```python
from build123d import *

# Parameters (mm, degrees)
BOX_W               = 29
BOX_H               = 73
BOX_DEPTH           = 10
BOX_PLACEMENT_ANGLE = 13
PAD_DEPTH           = 27.6


with BuildPart() as cube:
    # Box → Box (new body)
    with BuildSketch(Plane.XY):
        with Locations((14.5, 36.5)):
            Rectangle(BOX_W, BOX_H)
    extrude(amount=BOX_DEPTH)


with BuildPart() as cube_1:
    # Box placement: moved
    add(cube.part.moved(Location((46, -5, -10))).rotate(Axis((46, -5, -10), (0, -1, 0)), BOX_PLACEMENT_ANGLE))


with BuildPart() as cutted_flask:
    # Sketch → Pad (new body)
    with BuildSketch(Plane.XY):
        with BuildLine():
            ThreePointArc((2.776495, 50.1), (0.813217, 49.286783), (0, 47.323505))
            Line((0, 2.776495), (0, 47.323505))
            ThreePointArc((0, 2.776495), (0.813217, 0.813217), (2.776495, 0))
            Line((45.947206, 0), (2.776495, 0))
            ThreePointArc((45.947206, 0), (47.381198, 0.172613), (48.733265, 0.680592))
            Line((71.324311, 12.41834), (48.733265, 0.680592))
            ThreePointArc((71.324311, 12.41834), (71.817845, 12.880043), (72, 13.530861))
            Line((72, 25.05), (72, 13.530861))
            Line((72, 25.05), (72, 36.102443))
            ThreePointArc((72, 36.102443), (71.822776, 36.745073), (71.341206, 37.206021))
            Line((71.341206, 37.206021), (48.765787, 49.376307))
            ThreePointArc((48.765787, 49.376307), (47.376999, 49.916284), (45.898298, 50.1))
            Line((2.776495, 50.1), (45.898298, 50.1))
        make_face()
    extrude(amount=PAD_DEPTH)

    # Cut: cut Cube
    add(cube_1.part, mode=Mode.SUBTRACT)


solid = cutted_flask.part
```
Could you check a few things on this model? Use its own coordinates, in mm. Round coordinates to 2 decimals unless told otherwise and drop trailing zeros. Loops run counter-clockwise (first coordinate to the right, second up) from the corner with the lowest first, then second, coordinate; pieces in that order, holes last. Notation, with made-up numbers: (69.5, 27) - (101.5, 27) arc R24 ccw to (101.5, 64) - close; hole circle Ø5 at (0, 15). An arc over 180 degrees is marked (long way). Answer in a Markdown table with one row per item. Add a question column.
(1) If we section it at A-A (z = 25.5): Please give me the cut outline in (x, y), plus the area to 3 significant figures.
(2) I need wall thicknesses on line 1 along Y through (x, z) = (46, 22.5); line 2 along Y through (x, z) = (48.5, 11.75); line 3 along Z through (x, y) = (45, 13). Which ranges of each line are inside material? Lowest first, please.
(3) If we section it at D-D (y = 10): Please give me the cut outline in (x, z).
(4) If we section it at C-C (x = 67): Please give me the cut outline in (y, z), plus the area to 3 significant figures.
(5) If we section it at B-B (y = 33): Please give me the cut outline in (x, z).
(6) I'm going to push flat-ended pins straight in: pin 1 (1.5 mm diameter, centred on y = 44, z = 5, fed in from +X); pin 2 (6 mm diameter, centred on x = 48, y = 31, fed in from -Z). Where does each tip first touch, or does it pass through?
Model answer:
| question | item | result |
|---|---|---|
| 1 | outline | (0, 2.78) arc R2.78 ccw to (2.78, 0) - (45.95, 0) arc R6.04 ccw to (48.73, 0.68) - (71.32, 12.42) arc R1.25 ccw to (72, 13.53) - (72, 36.1) arc R1.25 ccw to (71.34, 37.21) - (48.77, 49.38) arc R6.04 ccw to (45.9, 50.1) - (2.78, 50.1) arc R2.78 ccw to (0, 47.32) - close |
| 1 | area | 3,280 mm² |
| 2 | line 1 | y = 0 to 50.1 |
| 2 | line 2 | y = 0.57 to 49.51 |
| 2 | line 3 | z = 0.03 to 27.6 |
| 3 | outline | (0, 0) - (44.86, 0) - (66.67, 5.04) - (66.67, 27.6) - (0, 27.6) - close |
| 4 | outline | (10.17, 5.11) - (39.55, 5.11) - (39.55, 27.6) - (10.17, 27.6) - close |
| 4 | area | 661 mm² |
| 5 | outline | (0, 0) - (44.86, 0) - (72, 6.27) - (72, 27.6) - (0, 27.6) - close |
| 6 | pin 1 | stops at x = 60.13 |
| 6 | pin 2 | stops at z = 0.03 |
